```python
from build123d import *

# Parameters (mm, degrees)
F1_DEPTH  = 114.3
F2_R      = 19.05
F3_DEPTH  = 25.4
F4_R      = 6.35
F5_DEPTH  = 12.7
F6_R      = 3.175
F7_DEPTH  = 12.7
F7_FACE_R = 3.175
F8_DEPTH  = 25.4
F9_R      = 9.525
F10_DEPTH = 19.05


with BuildPart() as f1:
    # F0 (on Front) → F1 (new body)
    with BuildSketch(Plane.XZ):
        with BuildLine():
            Line((139.7, 0), (38.1, 0))
            ThreePointArc((38.1, 0), (11.159232, -11.159232), (0, -38.1))
            Line((0, -38.1), (0, -69.85))
            Line((0, -69.85), (139.7, -69.85))
            ThreePointArc((139.7, -69.85), (148.680256, -66.130256), (152.4, -57.15))
            Line((152.4, -57.15), (152.4, -12.7))
            ThreePointArc((152.4, -12.7), (148.680256, -3.719744), (139.7, 0))
        make_face()
    extrude(amount=F1_DEPTH)

    # F2 (on face) → F3 (join)
    with BuildSketch(Plane.XZ.offset(114.3)):
        with Locations((126.039833, -34.362618)):
            Circle(F2_R)
    extrude(amount=F3_DEPTH)

    # F4 (on face) → F5 (join)
    with BuildSketch(Plane(origin=(0, 0, -69.85), x_dir=(1, 0, 0), z_dir=(0, 0, -1))):
        with Locations((7.622689, 107.050315)):
            Circle(F4_R)
    extrude(amount=F5_DEPTH)

    # F6 (on face) → F7 (join)
    with BuildSketch(Plane.YZ.offset(152.4)):
        with Locations((-127.194032, -32.0675)):
            Circle(F6_R)
    extrude(amount=-F7_DEPTH)

    # F7_face (on face) → F8 (join)
    with BuildSketch(Plane(origin=(152.4, -127.194032, -32.0675), x_dir=(0, 1, 0), z_dir=(1, 0, 0))):
        Circle(F7_FACE_R)
    extrude(amount=F8_DEPTH)

    # F9 (on face) → F10 (join)
    with BuildSketch(Plane(origin=(0, 0, 0), x_dir=(-1, 0, 0), z_dir=(0, 1, 0))):
        with Locations((-118.092358, -32.808334)):
            Circle(F9_R)
        with Locations((-36.353748, -33.302221)):
            Circle(F9_R)
    extrude(amount=F10_DEPTH)


solid = f1.part
```
CAD build for the part. Positions are in the model's coordinates, mm. A direction names the side the tool comes from. Give positions to 0.01 mm unless a question says otherwise; leave off trailing zeros. Write each loop counter-clockwise with the first axis right and the second up, starting at its lowest first coordinate (ties: lowest second). Pieces come first, ordered by that corner, then holes. Notation, with made-up numbers: M 87.25,-11.5 L 137.25,-11.5 A27 cw 137.25,7.5 Z; hole C 52,39.5 d11. An arc over 180 degrees is marked long. Return JSON: item names as keys, results as strings. Group by question number.
(1) Drill centre lines: L1, parallel to Y at x = 105, z = -48.5; L2, parallel to Z at x = 61, y = -74.5; L3, parallel to Y at x = 134, z = -40.5. Where is each one in solid material? Low to high. Write a range as [from, to].
(2) Flat gauge pins, fed straight in: pin 1 Ø3 at (x, z) = (24.5, -48) entering from +Y; pin 2 Ø1.5 at (x, y) = (117.5, -34.5) entering from -Z; pin 3 Ø1 at (x, y) = (23.5, -85) entering from +Z. Where does each tip first touch, or does it go through?
(3) Band-saw the part on C-C (x = 134). Give the cut face in (y, z), and give its area (3 significant figures).
(4) 3-axis set-ups, long thin cutter, end or side, ignore diameter. For faces 5 (the face through (177.8, -127, -32)), 6 (the face through (75, 0, -34)), 7 (the face through (6.796, -113.346, -76.111)), 8 (the face through (152.4, -56, -35)), 9 (the face through (118, 19.05, -33)): which of +Z, -Z, +X, -X, +Y, -Y reach the whole face in a straight line?
(5) Mould opens along X. For faces 1 (the face through (126, -139.7, -34)), 2 (the face through (148.58, -56.35, -66.23)), 3 (the face through (43.91, 9.39, -39.1)), 4 (the face through (127.61, 9.39, -32.39)) say: pulls with the +X half, pulls with the -X half, needs draft (parallel to the pull), parting line crosses it, or undercut.
(6) Band-saw the part on B-B (z = -18.5). Give the cut face in (x, y).
(7) Band-saw the part on D-D (y = -104.5). Give the cut face in (x, z).
(8) Band-saw the part on A-A (y = -71.5). Give the cut face in (x, z), and give its area (3 significant figures).
Entries:
{
 "1": {"L1": "y = [-114.3, 0]", "L2": "z = [-69.85, 0]", "L3": "y = [-139.7, 0]"},
 "2": {"pin 1": "stops at y = 0", "pin 2": "stops at z = -69.85", "pin 3": "stops at z = -2.71"},
 "3": {"outline": "M -139.7,-51.67 L -114.3,-51.67 L -114.3,-69.85 L 0,-69.85 L 0,0 L -114.3,0 L -114.3,-17.06 L -139.7,-17.06 Z", "area": "8,860 mm^2"},
 "4": {"face 5": "+Z, -Z, +X, +Y, -Y", "face 6": "+Y", "face 7": "-Z", "face 8": "+Z, -Z, +X, +Y", "face 9": "+Z, -Z, +X, -X, +Y"},
 "5": {"face 1": "needs draft", "face 2": "pulls with the +X half", "face 3": "undercut", "face 4": "undercut"},
 "6": {"outline": "M 5.43,-114.3 L 115.49,-114.3 L 115.49,-139.7 L 136.59,-139.7 L 136.59,-114.3 L 152.4,-114.3 L 152.4,0 L 5.43,0 Z"},
 "7": {"outline": "M 0,-69.85 L 1.81,-69.85 L 1.81,-82.55 L 13.44,-82.55 L 13.44,-69.85 L 139.7,-69.85 A12.7 ccw 152.4,-57.15 L 152.4,-12.7 A12.7 ccw 139.7,0 L 38.1,0 A38.1 ccw 0,-38.1 Z"},
 "8": {"outline": "M 0,-69.85 L 139.7,-69.85 A12.7 ccw 152.4,-57.15 L 152.4,-12.7 A12.7 ccw 139.7,0 L 38.1,0 A38.1 ccw 0,-38.1 Z", "area": "10,300 mm^2"}
}
